```python
from build123d import *

# Parameters (mm, degrees)
SKETCH1_W           = 7.62
SKETCH1_H           = 7.62
BOSS_EXTRUDE1_DEPTH = 19.05
SKETCH2_W           = 6.032118198
SKETCH2_H           = 12.495149586
CUT_EXTRUDE1_DEPTH  = 8.62
SKETCH4_W           = 7.62
SKETCH4_H           = 19.05
BOSS_EXTRUDE3_DEPTH = 0.762


with BuildPart() as part:
    # Sketch1 → Boss-Extrude1 (new body)
    with BuildSketch(Plane(origin=(0, 0, 0), x_dir=(1, 0, 0), z_dir=(0, 1, 0))):
        Rectangle(SKETCH1_W, SKETCH1_H)
    extrude(amount=BOSS_EXTRUDE1_DEPTH)

    # Sketch2 → Cut-Extrude1 (cut, through all)
    with BuildSketch(Plane.XY.offset(3.81)):
        with Locations((0, 9.525)):
            Rectangle(SKETCH2_W, SKETCH2_H)
    extrude(amount=-CUT_EXTRUDE1_DEPTH, mode=Mode.SUBTRACT)

    # Sketch4 → Boss-Extrude3 (add)
    with BuildSketch(Plane.XY.offset(3.81)):
        with Locations((0, 9.525)):
            Rectangle(SKETCH4_W, SKETCH4_H)
    extrude(amount=-BOSS_EXTRUDE3_DEPTH)


solid = part.part
```
Verification items for the finished model (mm, model axes). A direction names the side the tool comes from. Coordinates: 2 decimals unless noted, no trailing zeros. Loops run counter-clockwise (first coordinate to the right, second up) from the corner with the lowest first, then second, coordinate; pieces in that order, holes last. Notation, with made-up numbers: (48.25, 37.5) - (83.25, 37.5) arc R22 ccw to (83.25, 53.5) - close; hole circle Ø7 at (54.5, 37). An arc over 180 degrees is marked (long way). Return JSON: item names as keys, results as strings.
1. Go/stop test with a flat-tipped pin: pin 1 (3 mm diameter, centred on x = 1, y = 10, fed in from -Z). Record where the tip stops, or that it passes through.
Established:
{"pin 1": "stops at z = 3.05"}
2. Thickness scan on L1, parallel to X at y = 15.5, z = -0.75; L2, parallel to Y at x = -1.5, z = -0.5; L3, parallel to Z at x = -2.5, y = 11.75. Record the ranges inside material, lowest first.
Established:
{"L1": "x = -3.81 to -3.02, 3.02 to 3.81", "L2": "y = 0 to 3.28, 15.77 to 19.05", "L3": "z = 3.05 to 3.81"}
3. Section check A-A, the plane z = 0.75. Record the boundary of the cut face in (x, y), then the cut area to 3 significant figures.
Established:
{"outline": "(-3.81, 0) - (3.81, 0) - (3.81, 19.05) - (-3.81, 19.05) - close; hole (-3.02, 3.28) - (3.02, 3.28) - (3.02, 15.77) - (-3.02, 15.77) - close", "area": "69.8 mm2"}
4. Section check C-C, the plane y = 12.5. Record the boundary of the cut face in (x, z), then the cut area to 3 significant figures.
Established:
{"outline": "(-3.81, -3.81) - (-3.02, -3.81) - (-3.02, 3.05) - (3.02, 3.05) - (3.02, -3.81) - (3.81, -3.81) - (3.81, 3.81) - (-3.81, 3.81) - close", "area": "16.7 mm2"}
5. Mould release check, pull along Y, two halves, no side actions. Record for faces 3 (the flat face through (-3.016, 9, 0)), 4 (the flat face through (0, 0, 0)), 5 (the flat face through (3.016, 9, 0)), 6 (the flat face through (-3.81, 9, 0)): +Y half, -Y half, draft (parallel to the pull), parting line (faces both ways), or undercut.
Established:
{"face 3": "undercut", "face 4": "-Y half", "face 5": "undercut", "face 6": "draft"}
6. Tool access check on faces 1 (the flat face through (0, 9, 3.81)), 2 (the flat face through (0, 3.277, 0)). Record the directions out of +Z, -Z, +X, -X, +Y, -Y that give a thin tool (end or side, any length) a straight path to the whole face; none if there is none.
Established:
{"face 1": "+Z, +X, -X, +Y, -Y", "face 2": "-Z"}
7. Section check B-B, the plane x = 2. Record the boundary of the cut face in (y, z).
Established:
{"outline": "(0, -3.81) - (3.28, -3.81) - (3.28, 3.05) - (15.77, 3.05) - (15.77, -3.81) - (19.05, -3.81) - (19.05, 3.81) - (0, 3.81) - close"}
